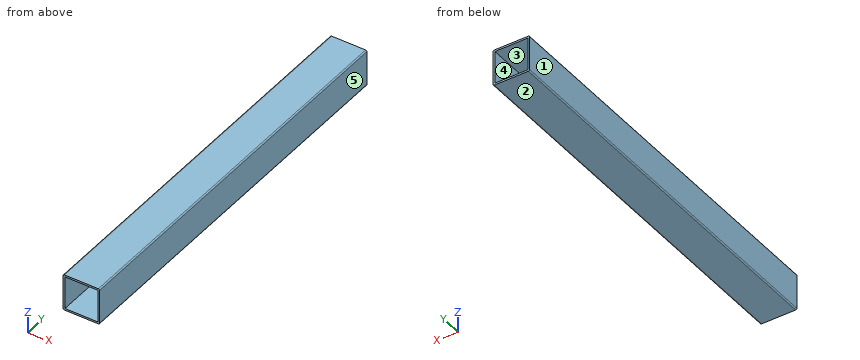
```python
from build123d import *

# Parameters (mm, degrees)
SKETCH1_W           = 54
SKETCH1_H           = 54
BOSS_EXTRUDE1_DEPTH = 650


with BuildPart() as part:
    # Sketch1 → Boss-Extrude1 (new body)
    with BuildSketch(Plane(origin=(0, 0, 0), x_dir=(1, 0, 0), z_dir=(0, 1, 0))):
        with BuildLine():
            Line((2, 0), (58, 0))
            ThreePointArc((58, 0), (59.414213562, 0.585786438), (60, 2))
            Line((60, 2), (60, 58))
            ThreePointArc((60, 58), (59.414213562, 59.414213562), (58, 60))
            Line((58, 60), (2, 60))
            ThreePointArc((2, 60), (0.585786438, 59.414213562), (0, 58))
            Line((0, 58), (0, 2))
            ThreePointArc((0, 2), (0.585786438, 0.585786438), (2, 0))
        make_face()
        with Locations((30, 30)):
            Rectangle(SKETCH1_W, SKETCH1_H, mode=Mode.SUBTRACT)
    extrude(amount=BOSS_EXTRUDE1_DEPTH)


solid = part.part
```
Input: part model. Units: mm. Frame: model coordinates. Face numbers are marked on the shaded views. A direction names the side the tool comes from. Coordinates: 2 decimals unless noted, no trailing zeros. Write each loop counter-clockwise with the first axis right and the second up, starting at its lowest first coordinate (ties: lowest second). Pieces come first, ordered by that corner, then holes.
1) Set-up query: the marked faces 4 and 5. Return all of +Z, -Z, +X, -X, +Y, -Y with unobstructed straight access to the full face (end or side cutting, diameter ignored); none if empty.
2) Material intervals for line 1 along X through (y, z) = (216.5, -9); line 2 along Z through (x, y) = (51, 68.5), sorted ascending.
3) Section A-A on x = 11. Output: boundary loops of the cut face in (y, z), and give its area (3 significant figures).
4) Section B-B on z = -51. Output: boundary loops of the cut face in (x, y), and give its area (3 significant figures).
5) Mould query, pull axis X, two halves, no side actions, for the marked faces 1, 2 and 3. Classes: pulls with the +X half, pulls with the -X half, needs draft (parallel to the pull), parting line crosses it, or undercut.
6) Section C-C on y = 69. Output: boundary loops of the cut face in (x, z).
Check result:
1. face 4: +Y, -Y
1. face 5: +Z, -Z, +X, +Y, -Y
2. line 1: x = 0 to 3, 57 to 60
2. line 2: z = -60 to -57, -3 to 0
3. outline: (0, -60) - (650, -60) - (650, -57) - (0, -57) - close; (0, -3) - (650, -3) - (650, 0) - (0, 0) - close
3. area: 3,900 mm2
4. outline: (0, 0) - (3, 0) - (3, 650) - (0, 650) - close; (57, 0) - (60, 0) - (60, 650) - (57, 650) - close
4. area: 3,900 mm2
5. face 1: pulls with the -X half
5. face 2: needs draft
5. face 3: undercut
6. outline: (0, -58) arc R2 ccw to (2, -60) - (58, -60) arc R2 ccw to (60, -58) - (60, -2) arc R2 ccw to (58, 0) - (2, 0) arc R2 ccw to (0, -2) - close; hole (3, -57) - (57, -57) - (57, -3) - (3, -3) - close
